Can you work these out from the model? Positions are in its coordinate system, mm. A direction names the side the tool comes from. Coordinates: 2 decimals unless noted, no trailing zeros. Order: outer loops, then holes, each group sorted by start corner. A loop starts at its lowest first (then second) coordinate and runs counter-clockwise, first axis right, second up. Notation, with made-up numbers: (7, -25.75) -> (65, -25.75) arc R15 cw to (65, -19.75) -> close; hole circle Ø2 at (83.5, 55.5). An arc over 180 degrees is marked (long way). Return JSON: item names as keys, results as strings. Group by question number.
1) If I drill on probe 1 along X at (y, z) = (-33, -20); probe 2 along Z at (x, y) = (81, 7.5); probe 3 along Y at (x, z) = (-28, 4), over which ranges is the centre line in solid material (lowest first)? Write a range as from..to.
2) For pin 1 (6 mm diameter, centred on x = 161.5, y = -46, fed in from +Z); pin 2 (5 mm diameter, centred on x = 138, z = 44.5, fed in from -Y); pin 3 (1 mm diameter, centred on x = -37, y = -40, fed in from +Z), each with a flat end and sliding along its axis, tell me the tip position at first contact or that it passes through.
3) For faces 4 (the cylindrical face through (161.78, 47.33, -61.73)), 5 (the cylindrical face through (-434.571, 49.592, -11.012)), 6 (the flat face through (-345.515, 29, 25)), which set-ups out of +Z, -Z, +X, -X, +Y, -Y let a thin tool reach every point of the face, with its end or its side?
4) Thinking about a two-plate mould opening in X: for faces 1 (the flat face through (289.485, 29, -25)), 2 (the cylindrical face through (-81.53, -23.84, 75.71)), 3 (the flat face through (-447.115, -1, -1)), which applies, +X half, -X half, draft (parallel to the pull), parting line (faces both ways), or undercut?
5) If we section it at A-A, the plane x = -182.5: Please give me the cut outline in (y, z) (3 decimals).
from build123d import *


# Not quite as in the source:
# - a fillet or chamfer that OpenCascade refuses, or shapes differently, is made with other operations: its cross-section is extruded or revolved along the edge and cut away or added


with BuildPart() as f1:
    # F0 (on Front) → F1 (revolve)
    with BuildSketch(Plane.XZ):
        with BuildLine():
            Line((-447.1154779911, 50.8), (-447.1154779911, 0))
            Line((-447.1154779911, 0), (391.0845220089, 0))
            Line((391.0845220089, 0), (391.0845220089, 50.8))
            Line((391.0845220089, 50.8), (365.6845220089, 50.8))
            Line((365.6845220089, 50.8), (365.6845220089, 38.1))
            Line((365.6845220089, 38.1), (289.4845220089, 38.1))
            Line((289.4845220089, 38.1), (289.4845220089, 50.8))
            ThreePointArc((289.4845220089, 50.8), (248.5849137461, 56.3889737285), (213.2845220089, 77.7875))
            Line((213.2845220089, 77.7875), (111.6845220089, 77.7875))
            Line((111.6845220089, 77.7875), (111.6845220089, 79.375))
            Line((111.6845220089, 79.375), (-269.3154779911, 79.375))
            ThreePointArc((-269.3154779911, 79.375), (-304.4294339656, 57.1247159319), (-345.5154779911, 50.8))
            Line((-345.5154779911, 50.8), (-345.5154779911, 38.1))
            Line((-345.5154779911, 38.1), (-421.7154779911, 38.1))
            Line((-421.7154779911, 38.1), (-421.7154779911, 50.8))
            Line((-421.7154779911, 50.8), (-447.1154779911, 50.8))
        make_face()
    revolve(axis=Axis((-28.0154779911, 0, 0), (1, 0, 0)))

    # F2: chamfer of 1.5875 on 8 edges, made by hand

    # F2_s1 → F2_t2 (revolve, cut)
    with BuildSketch(Plane.XZ):
        Polygon((-445.5279779911, 50.8), (-447.1154779911, 49.2125), (-447.1154779911, 50.8), align=None)
    revolve(axis=Axis((-447.1154779911, 0, 0), (1, 0, 0)), mode=Mode.SUBTRACT)

    # F2_s3 → F2_t4 (revolve, cut)
    with BuildSketch(Plane.XZ):
        Polygon((-421.7154779911, 49.2125), (-423.3029779911, 50.8), (-421.7154779911, 50.8), align=None)
    revolve(axis=Axis((-421.7154779911, 0, 0), (1, 0, 0)), mode=Mode.SUBTRACT)

    # F2_s5 → F2_t6 (revolve, cut)
    with BuildSketch(Plane.XZ):
        with BuildLine():
            Line((-343.8691410317, 50.7255652721), (-345.5154779911, 49.1391559736))
            Line((-345.5154779911, 49.1391559736), (-345.5154779911, 50.8))
            ThreePointArc((-345.5154779911, 50.8), (-344.6706324334, 50.7584599548), (-343.8691410317, 50.7255652721))
        make_face()
    revolve(axis=Axis((-345.5154779911, 0, 0), (1, 0, 0)), mode=Mode.SUBTRACT)

    # F2_s7 → F2_t8 (revolve, cut)
    with BuildSketch(Plane.XZ):
        Polygon((391.0845220089, 49.2125), (389.4970220089, 50.8), (391.0845220089, 50.8), align=None)
    revolve(axis=Axis((391.0845220089, 0, 0), (1, 0, 0)), mode=Mode.SUBTRACT)

    # F2_s9 → F2_t10 (revolve, cut)
    with BuildSketch(Plane.XZ):
        Polygon((367.2720220089, 50.8), (365.6845220089, 49.2125), (365.6845220089, 50.8), align=None)
    revolve(axis=Axis((365.6845220089, 0, 0), (1, 0, 0)), mode=Mode.SUBTRACT)

    # F2_s11 → F2_t12 (revolve, cut)
    with BuildSketch(Plane.XZ):
        with BuildLine():
            Line((289.4845220089, 49.1134387616), (287.8140491072, 50.6987689315))
            ThreePointArc((287.8140491072, 50.6987689315), (288.6278622062, 50.7446363641), (289.4845220089, 50.8))
            Line((289.4845220089, 50.8), (289.4845220089, 49.1134387616))
        make_face()
    revolve(axis=Axis((289.4845220089, 0, 0), (1, 0, 0)), mode=Mode.SUBTRACT)

    # F2_s13 → F2_t14 (revolve, cut)
    with BuildSketch(Plane.XZ):
        with BuildLine():
            Line((213.7373414064, 77.3686138432), (212.6628657503, 77.7875))
            Line((212.6628657503, 77.7875), (213.2845220089, 77.7875))
            ThreePointArc((213.2845220089, 77.7875), (213.5323086027, 77.5576500764), (213.7373414064, 77.3686138432))
        make_face()
    revolve(axis=Axis((213.2845220089, 0, 0), (1, 0, 0)), mode=Mode.SUBTRACT)

    # F2_s15 → F2_t16 (revolve, cut)
    with BuildSketch(Plane.XZ):
        with BuildLine():
            Line((-269.7732330498, 78.9331655442), (-268.6743214469, 79.375))
            Line((-268.6743214469, 79.375), (-269.3154779911, 79.375))
            ThreePointArc((-269.3154779911, 79.375), (-269.5651837952, 79.1332927093), (-269.7732330498, 78.9331655442))
        make_face()
    revolve(axis=Axis((-269.3154779911, 0, 0), (1, 0, 0)), mode=Mode.SUBTRACT)

    # F3: chamfer of 0.762 on 4 edges, made by hand

    # F3_s1 → F3_t2 (revolve)
    with BuildSketch(Plane.XZ):
        Polygon((111.6845220089, 78.5495), (112.4465220089, 77.7875), (111.6845220089, 77.7875), align=None)
    revolve(axis=Axis((111.6845220089, 0, 0), (1, 0, 0)))

    # F3_s3 → F3_t4 (revolve, cut)
    with BuildSketch(Plane.XZ):
        Polygon((110.9225220089, 79.375), (111.6845220089, 78.613), (111.6845220089, 79.375), align=None)
    revolve(axis=Axis((111.6845220089, 0, 0), (1, 0, 0)), mode=Mode.SUBTRACT)

    # F3_s5 → F3_t6 (revolve, cut)
    with BuildSketch(Plane.XZ):
        Polygon((212.5195839157, 77.7875), (212.7963616249, 77.7354564069), (212.6628657503, 77.7875), align=None)
    revolve(axis=Axis((212.6628657503, 0, 0), (1, 0, 0)), mode=Mode.SUBTRACT)


solid = f1.part
Result sheet:
{
 "1": {"probe 1": "x = -447.12..-421.72, -345.52..289.48, 365.68..391.08", "probe 2": "z = -79.02..79.02", "probe 3": "y = -79.27..79.27"},
 "2": {"pin 1": "stops at z = 64.82", "pin 2": "stops at y = -65.47", "pin 3": "stops at z = 68.85"},
 "3": {"face 4": "+X", "face 5": "-X", "face 6": "none"},
 "4": {"face 1": "undercut", "face 2": "draft", "face 3": "-X half"},
 "5": {"outline": "circle Ø158.75 at (0, 0)"}
}
